```python
from build123d import *

# Parameters (mm, degrees)
SKETCH1_R                               = 23
SKETCH1_R_2                             = 1.5
BOSS_EXTRUDE1_DEPTH                     = 12
SKETCH2_R                               = 20
SKETCH2_R_2                             = 12.7
CUT_EXTRUDE1_DEPTH                      = 6
FILLET1_R                               = 3
CBORE_FOR_M5_HEX_HEAD_BOLT1_D           = 5
CBORE_FOR_M5_HEX_HEAD_BOLT1_CBORE_D     = 8.5
CBORE_FOR_M5_HEX_HEAD_BOLT1_CBORE_DEPTH = 5.5
SKETCH5_R                               = 8.5
CUT_EXTRUDE2_DEPTH                      = 2


with BuildPart() as part:
    # Sketch1 → Boss-Extrude1 (new body)
    with BuildSketch(Plane.XY):
        Circle(SKETCH1_R)
        with Locations((0, 16.3)):
            Circle(SKETCH1_R_2, mode=Mode.SUBTRACT)
        with Locations((14.116214082, 8.15)):
            Circle(SKETCH1_R_2, mode=Mode.SUBTRACT)
        with Locations((14.116214082, -8.15)):
            Circle(SKETCH1_R_2, mode=Mode.SUBTRACT)
        with Locations((0, -16.3)):
            Circle(SKETCH1_R_2, mode=Mode.SUBTRACT)
        with Locations((-14.116214082, -8.15)):
            Circle(SKETCH1_R_2, mode=Mode.SUBTRACT)
        with Locations((-14.116214082, 8.15)):
            Circle(SKETCH1_R_2, mode=Mode.SUBTRACT)
    extrude(amount=BOSS_EXTRUDE1_DEPTH)

    # Sketch2 → Cut-Extrude1 (cut)
    with BuildSketch(Plane(origin=(0, 0, 0), x_dir=(-1, 0, 0), z_dir=(0, 0, -1))):
        Circle(SKETCH2_R)
        Circle(SKETCH2_R_2, mode=Mode.SUBTRACT)
    extrude(amount=-CUT_EXTRUDE1_DEPTH, mode=Mode.SUBTRACT)

    # Fillet1
    fillet1_edges = [part.edges().sort_by_distance(p)[0] for p in [
        (-23, 0, 12),
    ]]
    fillet(fillet1_edges, radius=FILLET1_R)

    # CBORE for M5 Hex Head Bolt1 (through all)
    with Locations(Plane.XY.offset(12)):
        with Locations((0, 0)):
            CounterBoreHole(CBORE_FOR_M5_HEX_HEAD_BOLT1_D / 2, CBORE_FOR_M5_HEX_HEAD_BOLT1_CBORE_D / 2, CBORE_FOR_M5_HEX_HEAD_BOLT1_CBORE_DEPTH)

    # Sketch5 → Cut-Extrude2 (cut)
    with BuildSketch(Plane(origin=(0, 0, 0), x_dir=(-1, 0, 0), z_dir=(0, 0, -1))):
        Circle(SKETCH5_R)
    extrude(amount=-CUT_EXTRUDE2_DEPTH, mode=Mode.SUBTRACT)


solid = part.part
```
For this review, take the finished solid that the model builds, in its own axes (mm). A direction names the side the tool comes from. Coordinates: 2 decimals unless noted, no trailing zeros. Loops run counter-clockwise (first coordinate to the right, second up) from the corner with the lowest first, then second, coordinate; pieces in that order, holes last. Notation, with made-up numbers: (-28, 68) -> (31, 68) arc R25 cw to (31, 103) -> close; hole circle Ø9 at (-10, -5.5). An arc over 180 degrees is marked (long way). Return JSON: item names as keys, results as strings. Group by question number.
(1) Consider section B-B, the plane z = 7.75. Give the boundary of the cut face in (x, y), plus the area to 3 significant figures.
(2) To check wall thickness, follow L1, parallel to Y at x = 0, z = 8.25; L2, parallel to Y at x = 0, z = 4.75; L3, parallel to X at y = -2, z = 2.5. State the ranges of each line that lie inside material, in increasing order.
(3) For pin 1 Ø3.5 at (x, y) = (14.12, -8.15) entering from -Z; pin 2 Ø2.5 at (x, y) = (2, -1) entering from +Z; pin 3 Ø13.5 at (x, y) = (0, 0) entering from +Z; pin 4 Ø1 at (x, z) = (-13.5, 9.5) entering from +Y, all flat-tipped, find the tip position at first contact; note any pin that passes through.
(4) Consider section C-C, the plane y = 0. Give the boundary of the cut face in (x, z), plus the area to 3 significant figures.
(5) Consider section A-A, the plane x = 0. Count the separate pieces of the cut face and the enclosed holes in it, plus the area to 3 significant figures.
(6) Consider section D-D, the plane z = 3.25. Give the boundary of the cut face in (x, y), plus the area to 3 significant figures.
(7) Mouldability with a two-part tool opening along X and no side actions: class faces 4 (the flat face through (0, 5, 12)), 5 (the cylindrical face through (15.547, 8.601, 8.958)), 6 (the cylindrical face through (-2.994, 22.804, 4.437)) as pulls with the +X half, pulls with the -X half, needs draft (parallel to the pull), parting line crosses it, or undercut.
(8) Tool access review of faces 1 (the cylindrical face through (2.75, -12.4, 2.96)), 2 (the flat face through (2, -2, 6.5)), 3 (the cylindrical face through (-13.31, 9.415, 8.958)): name each direction out of +Z, -Z, +X, -X, +Y, -Y from which nothing blocks a thin tool from reaching the whole face with its end or side.
Results below:
{
 "1": {"outline": "circle Ø46 at (0, 0); hole circle Ø3 at (-14.12, -8.15); hole circle Ø3 at (-14.12, 8.15); hole circle Ø8.5 at (0, 0); hole circle Ø3 at (0, -16.3); hole circle Ø3 at (0, 16.3); hole circle Ø3 at (14.12, -8.15); hole circle Ø3 at (14.12, 8.15)", "area": "1,560 mm2"},
 "2": {"L1": "y = -23 to -17.8, -14.8 to -4.25, 4.25 to 14.8, 17.8 to 23", "L2": "y = -23 to -20, -12.7 to -2.5, 2.5 to 12.7, 20 to 23", "L3": "x = -22.91 to -19.9, -12.54 to -1.5, 1.5 to 12.54, 19.9 to 22.91"},
 "3": {"pin 1": "stops at z = 6", "pin 2": "stops at z = 6.5", "pin 3": "stops at z = 12", "pin 4": "stops at y = 18.93"},
 "4": {"outline": "(-23, 0) -> (-20, 0) -> (-20, 6) -> (-12.7, 6) -> (-12.7, 0) -> (-8.5, 0) -> (-8.5, 2) -> (-2.5, 2) -> (-2.5, 6.5) -> (-4.25, 6.5) -> (-4.25, 12) -> (-20, 12) arc R3 ccw to (-23, 9) -> close; (2.5, 2) -> (8.5, 2) -> (8.5, 0) -> (12.7, 0) -> (12.7, 6) -> (20, 6) -> (20, 0) -> (23, 0) -> (23, 9) arc R3 ccw to (20, 12) -> (4.25, 12) -> (4.25, 6.5) -> (2.5, 6.5) -> close", "area": "357 mm2"},
 "5": {"separate pieces": "4", "enclosed holes": "0", "area": "321 mm2"},
 "6": {"outline": "circle Ø46 at (0, 0); circle Ø25.4 at (0, 0); hole circle Ø40 at (0, 0); hole circle Ø5 at (0, 0)", "area": "892 mm2"},
 "7": {"face 4": "needs draft", "face 5": "undercut", "face 6": "parting line crosses it"},
 "8": {"face 1": "-Z", "face 2": "+Z", "face 3": "+Z, -Z"}
}
